For this review, take the finished solid that the model builds, in its own axes (mm). Round coordinates to 2 decimals unless told otherwise and drop trailing zeros. Order: outer loops, then holes, each group sorted by start corner. A loop starts at its lowest first (then second) coordinate and runs counter-clockwise, first axis right, second up. Notation, with made-up numbers: (35.25, 0.5) -> (68.25, 0.5) arc R18 cw to (68.25, 34.5) -> close; hole circle Ø1 at (2.5, -19.75). An arc over 180 degrees is marked (long way). Put each result on its own line as item: value. Start each with the question number.
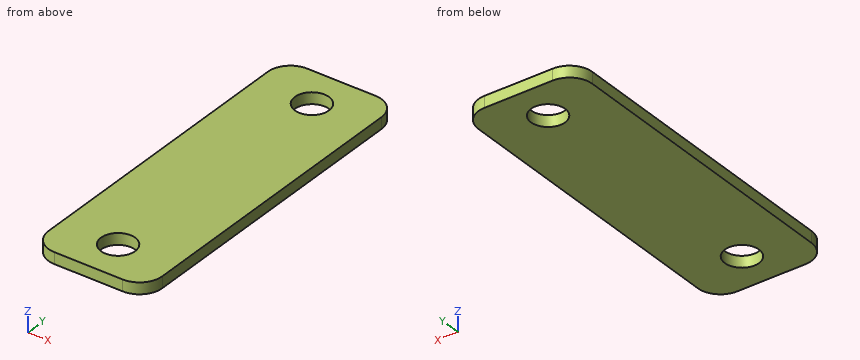
```python
from build123d import *

# Parameters (mm, degrees)
SKETCH_1_W          = 10
SKETCH_1_H          = 30
EXTRUDE_1_DEPTH     = 0.5
SKETCH_2_R          = 1.5
CUT_EXTRUDE_1_DEPTH = 10
FILLET_1_R          = 2


with BuildPart() as part:
    # 草图1 → 凸台-拉伸1 (new, symmetric)
    with BuildSketch(Plane.XY):
        Rectangle(SKETCH_1_W, SKETCH_1_H)
    extrude(amount=EXTRUDE_1_DEPTH, both=True)

    # 草图2 → 切除-拉伸1 (cut)
    with BuildSketch(Plane.XY.offset(0.5)):
        with Locations((0, 11.5)):
            Circle(SKETCH_2_R)
        with Locations((0, -11.5)):
            Circle(SKETCH_2_R)
    extrude(amount=-CUT_EXTRUDE_1_DEPTH, mode=Mode.SUBTRACT)

    # 圆角1
    fillet_1_edges = [part.edges().sort_by_distance(p)[0] for p in [
        (5, -15, 0),
        (-5, -15, 0),
        (-5, 15, 0),
        (5, 15, 0),
    ]]
    fillet(fillet_1_edges, radius=FILLET_1_R)


solid = part.part
```
Item 1: Consider section A-A, the plane x = 0. Write out the cut boundary in (y, z).
Item 2: For L1, parallel to Y at x = 0, z = -0.05; L2, parallel to Y at x = 1, z = 0.2, list the stretches that pass through material, from the lowest coordinate up.
Item 3: Consider section B-B, the plane y = -11.5. Write out the cut boundary in (x, z), plus the area to 3 significant figures.
Item 4: Consider section C-C, the plane z = -0.3. Write out the cut boundary in (x, y), plus the area to 3 significant figures.
Evaluation:
1. outline: (-15, -0.5) -> (-13, -0.5) -> (-13, 0.5) -> (-15, 0.5) -> close; (-10, -0.5) -> (10, -0.5) -> (10, 0.5) -> (-10, 0.5) -> close; (13, -0.5) -> (15, -0.5) -> (15, 0.5) -> (13, 0.5) -> close
2. L1: y = -15 to -13, -10 to 10, 13 to 15
2. L2: y = -15 to -12.62, -10.38 to 10.38, 12.62 to 15
3. outline: (-5, -0.5) -> (-1.5, -0.5) -> (-1.5, 0.5) -> (-5, 0.5) -> close; (1.5, -0.5) -> (5, -0.5) -> (5, 0.5) -> (1.5, 0.5) -> close
3. area: 7.00 mm^2
4. outline: (-5, -13) arc R2 ccw to (-3, -15) -> (3, -15) arc R2 ccw to (5, -13) -> (5, 13) arc R2 ccw to (3, 15) -> (-3, 15) arc R2 ccw to (-5, 13) -> close; hole circle Ø3 at (0, -11.5); hole circle Ø3 at (0, 11.5)
4. area: 282 mm^2
